Could you check a few things on this model? Use its own coordinates, in mm. A direction names the side the tool comes from. Round coordinates to 2 decimals unless told otherwise and drop trailing zeros. Order: outer loops, then holes, each group sorted by start corner. A loop starts at its lowest first (then second) coordinate and runs counter-clockwise, first axis right, second up. Notation, with made-up numbers: (53, -20.75) -> (81, -20.75) arc R19 ccw to (81, 6.25) -> close; hole circle Ø3 at (-3.5, 6.25). An arc over 180 degrees is marked (long way). Put each result on its own line as item: value. Start each with the question number.
from build123d import *

# Parameters (mm, degrees)
BOSS_EXTRUDE1_DEPTH      = 4
SKETCH2_R                = 2.5
CUT_EXTRUDE1_DEPTH       = 22.9089023
SKETCH3_R                = 3.05
CUT_EXTRUDE2_DEPTH       = 2
CUT_EXTRUDE3_DEPTH       = 1.2
CUT_EXTRUDE5_DEPTH       = 0.7
CUT_EXTRUDE8_START       = -2
CUT_EXTRUDE8_DEPTH       = 2
BOSS_EXTRUDE3_DEPTH      = 2
BOSS_EXTRUDE4_DEPTH      = 1.9
CUT_EXTRUDE10_DEPTH      = 22.9089023
CUT_EXTRUDE10_DEPTH_BACK = 22.9089023
CUT_EXTRUDE11_DEPTH      = 23.360679775
CUT_EXTRUDE12_DEPTH      = 24.837994882
CUT_EXTRUDE12_DEPTH_BACK = 24.837994882
CHAMFER1_SIZE            = 1.75
CUT_EXTRUDE13_DEPTH      = 24.837994882
CUT_EXTRUDE14_DEPTH      = 21.155644371
CHAMFER2_SIZE            = 0.5


with BuildPart() as part:
    # Sketch1 → Boss-Extrude1 (new body)
    with BuildSketch(Plane(origin=(0, 0, 0), x_dir=(1, 0, 0), z_dir=(0, 1, 0))):
        with BuildLine():
            Line((-6.5, -20), (6.5, -20))
            Line((6.5, -20), (6.5, -4.663689527))
            ThreePointArc((6.5, -4.663689527), (8, 0), (6.5, 4.663689527))
            ThreePointArc((6.5, 4.663689527), (0, 8), (-6.5, 4.663689527))
            ThreePointArc((-6.5, 4.663689527), (-8, 0), (-6.5, -4.663689527))
            Line((-6.5, -4.663689527), (-6.5, -20))
        make_face()
    extrude(amount=-BOSS_EXTRUDE1_DEPTH)

    # Sketch2 → Cut-Extrude1 (cut, through all)
    with BuildSketch(Plane(origin=(0, 0, 0), x_dir=(1, 0, 0), z_dir=(0, 1, 0))):
        with Locations(Location((0, 0, 0), (0, 0, 270))):
            Circle(SKETCH2_R)
    extrude(amount=-CUT_EXTRUDE1_DEPTH, mode=Mode.SUBTRACT)

    # Sketch3 → Cut-Extrude2 (cut)
    with BuildSketch(Plane(origin=(0, 0, 0), x_dir=(1, 0, 0), z_dir=(0, 1, 0))):
        with Locations(Location((0, 0, 0), (0, 0, 270))):
            Circle(SKETCH3_R)
    extrude(amount=-CUT_EXTRUDE2_DEPTH, mode=Mode.SUBTRACT)

    # Sketch4 → Cut-Extrude3 (cut)
    with BuildSketch(Plane.XZ.offset(4)):
        Polygon((2.5, -5.75), (-2.5, -5.75), (-5.75, -2.5), (-5.75, 6.75), (-4.75, 6.75), (-4.75, 8.2), (-6.010373569, 10), (-6.5, 10), (-6.5, 10.699259012), (-6.5, 15), (6.5, 15), (6.5, 10.699259012), (6.5, 10), (6.5, 8.2), (4.75, 8.2), (4.75, 6.75), (5.75, 6.75), (5.75, -2.5), align=None)
    extrude(amount=-CUT_EXTRUDE3_DEPTH, mode=Mode.SUBTRACT)

    # Sketch6 → Cut-Extrude5 (cut)
    with BuildSketch(Plane.XZ.offset(2.8)):
        Polygon((6.5, 8.2), (6.5, 15), (-6.5, 15), (-6.5, 10.699259012), (-6.010373569, 10), (-4.75, 8.2), (-4.75, 6.2), (4.75, 6.2), (4.75, 8.2), align=None)
    extrude(amount=-CUT_EXTRUDE5_DEPTH, mode=Mode.SUBTRACT)

    # Sketch10 → Cut-Extrude8 (cut)
    with BuildSketch(Plane.XZ.offset(4).offset(CUT_EXTRUDE8_START)):
        with BuildLine():
            Line((-6.5, 4.663689527), (-6.5, -2.5))
            Line((-6.5, -2.5), (-7.599342077, -2.5))
            ThreePointArc((-7.599342077, -2.5), (-7.907431546, 1.213476964), (-6.5, 4.663689527))
        make_face()
        with BuildLine():
            Line((6.5, 4.663689527), (6.5, -2.5))
            Line((6.5, -2.5), (7.599342077, -2.5))
            ThreePointArc((7.599342077, -2.5), (7.907431546, 1.213476964), (6.5, 4.663689527))
        make_face()
    extrude(amount=CUT_EXTRUDE8_DEPTH, mode=Mode.SUBTRACT)

    # Sketch11 → Boss-Extrude3 (add)
    with BuildSketch(Plane.XZ.offset(4)):
        with BuildLine():
            Line((-0.75, -7.964766161), (-0.75, -5.75))
            Line((-0.75, -5.75), (-2.5, -5.75))
            Line((-2.5, -5.75), (-4.125, -4.125))
            Line((-4.125, -4.125), (-5.656854249, -5.656854249))
            ThreePointArc((-5.656854249, -5.656854249), (-3.404931672, -7.239229262), (-0.75, -7.964766161))
        make_face()
        with BuildLine():
            Line((0.75, -7.964766161), (0.75, -5.75))
            Line((0.75, -5.75), (2.5, -5.75))
            Line((2.5, -5.75), (4.125, -4.125))
            Line((4.125, -4.125), (5.656854249, -5.656854249))
            ThreePointArc((5.656854249, -5.656854249), (3.404931672, -7.239229262), (0.75, -7.964766161))
        make_face()
    extrude(amount=BOSS_EXTRUDE3_DEPTH)

    # Sketch14 → Boss-Extrude4 (add)
    with BuildSketch(Plane.XZ.offset(2.1)):
        Polygon((-4.75, 8.2), (-6.010373569, 10), (-6.5, 10), (-6.5, 15), (-4.75, 15), align=None)
    extrude(amount=BOSS_EXTRUDE4_DEPTH)

    # Sketch15 → Cut-Extrude10 (cut, two sides: drawn at the far end of the back side and taken through both)
    with BuildSketch(Plane.XZ.offset(4).offset(-CUT_EXTRUDE10_DEPTH_BACK)):
        Polygon((-6.5, 15), (-6.5, 8.2), (-4.75, 8.2), (-4.75, 15), (-3.5, 15), (-3.5, 20), (-6.5, 20), align=None)
        Polygon((6.5, 8.2), (4.75, 8.2), (4.75, 15), (3.5, 15), (3.5, 20), (6.5, 20), (6.5, 15), align=None)
    extrude(amount=CUT_EXTRUDE10_DEPTH + CUT_EXTRUDE10_DEPTH_BACK, mode=Mode.SUBTRACT)

    # Sketch16 → Cut-Extrude11 (cut, through all)
    with BuildSketch(Plane(origin=(0, 0, 0), x_dir=(1, 0, 0), z_dir=(0, 1, 0))):
        Polygon((-1.75, -15), (-4.75, -12), (-4.75, -15), (-3.5, -15), align=None)
        Polygon((4.75, -12), (4.75, -15), (1.75, -15), align=None)
    extrude(amount=-CUT_EXTRUDE11_DEPTH, mode=Mode.SUBTRACT)

    # Sketch17 → Cut-Extrude12 (cut, two sides: drawn at the far end of the back side and taken through both)
    with BuildSketch(Plane(origin=(3.5, 0, 0), x_dir=(0, 0, -1), z_dir=(1, 0, 0)).offset(-CUT_EXTRUDE12_DEPTH_BACK)):
        with BuildLine():
            Line((-16.25, -4), (-18.75, -4))
            ThreePointArc((-18.75, -4), (-17.5, -2.75), (-16.25, -4))
        make_face()
    extrude(amount=CUT_EXTRUDE12_DEPTH + CUT_EXTRUDE12_DEPTH_BACK, mode=Mode.SUBTRACT)

    # Chamfer1
    chamfer1_edges = [part.edges().sort_by_distance(p)[0] for p in [
        (-4.75, -1.05, 8.2),
        (4.75, -1.05, 8.2),
    ]]
    chamfer(chamfer1_edges, length=CHAMFER1_SIZE - 0.0001)  # a hair under: the kernel refuses the full size

    # Sketch18 → Cut-Extrude13 (cut, through all)
    with BuildSketch(Plane(origin=(3.5, 0, 0), x_dir=(0, 0, -1), z_dir=(1, 0, 0))):
        with BuildLine():
            Line((-18.75, -4), (-20, -4))
            Line((-20, -4), (-20, 0))
            Line((-20, 0), (-18.75, 0))
            Line((-18.75, 0), (-17.5, 0))
            Line((-17.5, 0), (-17.5, -2.75))
            ThreePointArc((-17.5, -2.75), (-18.383883476, -3.116116524), (-18.75, -4))
        make_face()
    extrude(amount=-CUT_EXTRUDE13_DEPTH, mode=Mode.SUBTRACT)

    # Sketch19 → Cut-Extrude14 (cut, through all)
    with BuildSketch(Plane(origin=(0, 0, 0), x_dir=(1, 0, 0), z_dir=(0, 1, 0))):
        Polygon((-3.5, -10.290482648), (-6.5, -6.006038628), (-6.5, -13.25), (-3.5, -13.25), align=None)
    extrude(amount=-CUT_EXTRUDE14_DEPTH, mode=Mode.SUBTRACT)

    # Chamfer2
    chamfer2_edges = [part.edges().sort_by_distance(p)[0] for p in [
        (0, 0, -3.05),
    ]]
    chamfer(chamfer2_edges, length=CHAMFER2_SIZE)


solid = part.part
1. If we section it at D-D, the plane z = 12.5: Please give me the cut outline in (x, y), then the cut area to 3 significant figures.
2. If we section it at B-B, the plane y = -5.1: Please give me the cut outline in (x, z) (3 decimals).
3. If we section it at C-C, the plane z = 0: Please give me the cut outline in (x, y).
4. If we section it at A-A, the plane x = 0: Please give me the cut outline in (y, z).
5. Thinking about a two-plate mould opening in X: for faces 1 (the face through (5, -3, 6.75)), 2 (the face through (-5.312, -1.528, 7.702)), 3 (the face through (0, -3.7, -5.75)), 4 (the face through (6.5, -2.4, 4.1)), which applies, +X half, -X half, draft (parallel to the pull), parting line (faces both ways), or undercut?
6. Which directions (+Z, -Z, +X, -X, +Y, -Y) give clear straight access to the entire face, cutting with the end or side of a thin tool? Please do faces 5 (the face through (0, -2.8, 3)), 6 (the face through (0, -4, 16)), 7 (the face through (-6.5, -3, 2)), 8 (the face through (3.23, -1.04, 13.52)), 9 (the face through (-0.75, -5, -7)).
7. I need wall thicknesses on L1, parallel to X at y = -2.35, z = 0; L2, parallel to X at y = -1.2, z = 0; L3, parallel to Y at x = -0.5, z = 10. Which ranges of each line are inside material? Lowest first, please.
8. For pin 1 Ø1 at (y, z) = (-3.5, 2) entering from +X; pin 2 Ø3 at (x, z) = (-6, 0.5) entering from -Y; pin 3 Ø1.5 at (y, z) = (-2.5, -3.5) entering from -X, each with a flat end and sliding along its axis, tell me the tip position at first contact or that it passes through.
Results below:
1. outline: (-3.5, -2.1) -> (4.25, -2.1) -> (4.25, 0) -> (-3.5, 0) -> close
1. area: 16.3 mm2
2. outline: (-5.657, -5.657) arc R8 ccw to (-0.75, -7.965) -> (-0.75, -5.75) -> (-2.5, -5.75) -> (-4.125, -4.125) -> close; (0.75, -7.965) arc R8 ccw to (5.657, -5.657) -> (4.125, -4.125) -> (2.5, -5.75) -> (0.75, -5.75) -> close
3. outline: (-8, -2) -> (-6.5, -2) -> (-6.5, -4) -> (-5.75, -4) -> (-5.75, -2.8) -> (-2.5, -2.8) -> (-2.5, -2) -> (-3.05, -2) -> (-3.05, -0.5) -> (-3.55, 0) -> (-8, 0) -> close; (2.5, -2.8) -> (5.75, -2.8) -> (5.75, -4) -> (6.5, -4) -> (6.5, -2) -> (8, -2) -> (8, 0) -> (3.55, 0) -> (3.05, -0.5) -> (3.05, -2) -> (2.5, -2) -> close
4. outline: (-4, -8) -> (0, -8) -> (0, -3.55) -> (-0.5, -3.05) -> (-2, -3.05) -> (-2, -2.5) -> (-2.8, -2.5) -> (-2.8, -5.75) -> (-4, -5.75) -> close; (-4, 15) -> (-2.1, 15) -> (-2.1, 6.2) -> (-2.8, 6.2) -> (-2.8, 2.5) -> (-2, 2.5) -> (-2, 3.05) -> (-0.5, 3.05) -> (0, 3.55) -> (0, 17.5) -> (-2.75, 17.5) arc R1.25 cw to (-4, 16.25) -> close
5. face 1: undercut
5. face 2: -X half
5. face 3: undercut
5. face 4: +X half
6. face 5: -Y
6. face 6: +Z, +X, -X, -Y
6. face 7: +Z, -X, -Y
6. face 8: +X, +Y, -Y
6. face 9: +Z, -Z, -Y
7. L1: -6.5 to -2.5, 2.5 to 6.5
7. L2: -8 to -3.05, 3.05 to 8
7. L3: -2.1 to 0
8. pin 1: x = 6.5
8. pin 2: y = -4
8. pin 3: x = -7.51
